Source: CAD feature listing. Evaluate the final solid. Frame: model axes, mm. Round coordinates to 2 decimals unless told otherwise and drop trailing zeros. Loops run counter-clockwise (first coordinate to the right, second up) from the corner with the lowest first, then second, coordinate; pieces in that order, holes last.
Item 1: Section query B-B on x = 12.7. Return loops of the section in (y, z).
Item 2: Section query D-D on y = 0.2. Give the number of separate pieces and of enclosed holes in the cut face, then the cut area to 3 significant figures.
Item 3: Pull-direction query (Z, two-part tool) for faces 1 (the cylindrical face through (-14.242, 0.296, -0.468)), 2 (the flat face through (9, 0, 0)), 3 (the cylindrical face through (-13.4, 0.3, 0.36)); classes: released by +Z, released by -Z, zero draft, split by the parting line, or undercut.
Item 4: Ray query, L1, parallel to X at y = 0.15, z = 0; L2, parallel to X at y = 0.1, z = -3.75; L3, parallel to X at y = 0.4, z = -8.89. Return the intervals inside material, ascending.
Item 5: Section query A-A on z = 0. Return loops of the section in (x, y).
Item 6: Section query C-C on z = 5. Return loops of the section in (x, y).
```python
from build123d import *

# Parameters (mm, degrees)
SKETCH1_R           = 0.7874
SKETCH1_R_2         = 8.5
SKETCH1_R_3         = 0.508
BOSS_EXTRUDE1_DEPTH = 0.6


with BuildPart() as part:
    # Sketch1 → Boss-Extrude1 (new body)
    # profile 1 of 3: a face of its own
    with BuildSketch(Plane(origin=(0, 0, 0), x_dir=(1, 0, 0), z_dir=(0, 1, 0))):
        with BuildLine():
            Line((9.991841672, -10.16), (9.991841672, 10.16))
            ThreePointArc((9.991841672, 10.16), (-14.25, 0), (9.991841672, -10.16))
        make_face()
        with Locations(Location((-8.980256121, -8.980256121, 0), (0, 0, 270))):
            Circle(SKETCH1_R, mode=Mode.SUBTRACT)
        with Locations(Location((0, -12.7, 0), (0, 0, 270))):
            Circle(SKETCH1_R, mode=Mode.SUBTRACT)
        with Locations(Location((8.980256121, -8.980256121, 0), (0, 0, 270))):
            Circle(SKETCH1_R, mode=Mode.SUBTRACT)
        with Locations(Location((-12.7, 0, 0), (0, 0, 270))):
            Circle(SKETCH1_R, mode=Mode.SUBTRACT)
        with Locations(Location((0, 0, 0), (0, 0, 270))):
            Circle(SKETCH1_R_2, mode=Mode.SUBTRACT)
        with Locations(Location((-8.980256121, 8.980256121, 0), (0, 0, 270))):
            Circle(SKETCH1_R, mode=Mode.SUBTRACT)
        with Locations(Location((0, 12.7, 0), (0, 0, 270))):
            Circle(SKETCH1_R, mode=Mode.SUBTRACT)
        with Locations(Location((8.980256121, 8.980256121, 0), (0, 0, 270))):
            Circle(SKETCH1_R, mode=Mode.SUBTRACT)
    # profile 2 of 3: a face of its own
    with BuildSketch(Plane(origin=(0, 0, 0), x_dir=(1, 0, 0), z_dir=(0, 1, 0))):
        with BuildLine():
            ThreePointArc((14.25, 0), (13.142416898, 5.508119288), (9.991841672, 10.16))
            Line((9.991841672, 10.16), (9.991841672, -10.16))
            ThreePointArc((9.991841672, -10.16), (13.142416898, -5.508119288), (14.25, 0))
        make_face()
        with Locations(Location((12.7, 0, 0), (0, 0, 270))):
            Circle(SKETCH1_R, mode=Mode.SUBTRACT)
    # profile 3 of 3: a face of its own
    with BuildSketch(Plane(origin=(0, 0, 0), x_dir=(1, 0, 0), z_dir=(0, 1, 0))):
        with BuildLine():
            Line((18.06, 10.16), (9.991841672, 10.16))
            ThreePointArc((9.991841672, 10.16), (13.142416898, 5.508119288), (14.25, 0))
            ThreePointArc((14.25, 0), (13.142416898, -5.508119288), (9.991841672, -10.16))
            Line((9.991841672, -10.16), (18.06, -10.16))
            Line((18.06, -10.16), (18.06, 10.16))
        make_face()
        with Locations(Location((16.79, -8.89, 0), (0, 0, 270))):
            Circle(SKETCH1_R_3, mode=Mode.SUBTRACT)
        with Locations(Location((16.79, -6.35, 0), (0, 0, 270))):
            Circle(SKETCH1_R_3, mode=Mode.SUBTRACT)
        with Locations(Location((16.79, -3.81, 0), (0, 0, 270))):
            Circle(SKETCH1_R_3, mode=Mode.SUBTRACT)
        with Locations(Location((16.79, -1.27, 0), (0, 0, 270))):
            Circle(SKETCH1_R_3, mode=Mode.SUBTRACT)
        with Locations(Location((16.79, 1.27, 0), (0, 0, 270))):
            Circle(SKETCH1_R_3, mode=Mode.SUBTRACT)
        with Locations(Location((16.79, 3.81, 0), (0, 0, 270))):
            Circle(SKETCH1_R_3, mode=Mode.SUBTRACT)
        with Locations(Location((16.79, 6.35, 0), (0, 0, 270))):
            Circle(SKETCH1_R_3, mode=Mode.SUBTRACT)
        with Locations(Location((16.79, 8.89, 0), (0, 0, 270))):
            Circle(SKETCH1_R_3, mode=Mode.SUBTRACT)
    extrude(amount=BOSS_EXTRUDE1_DEPTH)


solid = part.part
```
Data:
1. outline: (0, -10.16) - (0.6, -10.16) - (0.6, -0.79) - (0, -0.79) - close; (0, 0.79) - (0.6, 0.79) - (0.6, 10.16) - (0, 10.16) - close
2. separate pieces: 1
2. enclosed holes: 17
2. area: 493 mm2
3. face 1: split by the parting line
3. face 2: zero draft
3. face 3: undercut
4. L1: x = -14.25 to -13.49, -11.91 to -8.5, 8.5 to 11.91, 13.49 to 18.06
4. L2: x = -13.75 to -7.63, 7.63 to 16.29, 17.29 to 18.06
4. L3: x = -11.14 to -9.76, -8.2 to 8.2, 9.76 to 16.28, 17.3 to 18.06
5. outline: (-14.25, 0) - (-13.49, 0) - (-13.49, 0.6) - (-14.25, 0.6) - close; (-11.91, 0) - (-8.5, 0) - (-8.5, 0.6) - (-11.91, 0.6) - close; (8.5, 0) - (11.91, 0) - (11.91, 0.6) - (8.5, 0.6) - close; (13.49, 0) - (18.06, 0) - (18.06, 0.6) - (13.49, 0.6) - close
6. outline: (-13.34, 0) - (-6.87, 0) - (-6.87, 0.6) - (-13.34, 0.6) - close; (6.87, 0) - (18.06, 0) - (18.06, 0.6) - (6.87, 0.6) - close
